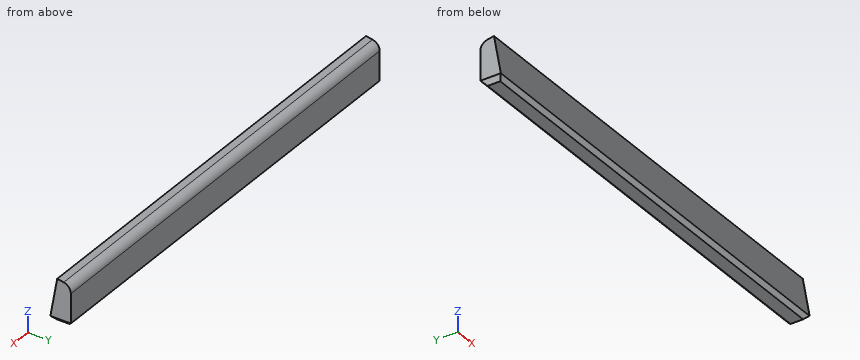
```python
from build123d import *

# Parameters (mm, degrees)
PAD001_DEPTH    = 26
CHAMFER002_SIZE = 0.5
FILLET001_R     = 1


with BuildPart() as part:
    # Sketch002 → Pad001 (new body, symmetric)
    with BuildSketch(Plane.YZ):
        Polygon((0, 0), (-1.575692, 0.277837), (-2.456946, -4.72), (0, -4.72), align=None)
    extrude(amount=PAD001_DEPTH, both=True)

    # Chamfer002
    chamfer002_edges = [part.edges().sort_by_distance(p)[0] for p in [
        (0, -2.456946, -4.72),
        (0, 0, -4.72),
        (-26, -1.228473, -4.72),
        (26, -1.228473, -4.72),
    ]]
    chamfer(chamfer002_edges, length=CHAMFER002_SIZE)

    # Fillet001
    fillet001_edges = [part.edges().sort_by_distance(p)[0] for p in [
        (0, 0, 0),
    ]]
    fillet(fillet001_edges, radius=FILLET001_R)


solid = part.part
```
Verification items for the finished model (mm, model axes). Coordinates: 2 decimals unless noted, no trailing zeros. Write each loop counter-clockwise with the first axis right and the second up, starting at its lowest first coordinate (ties: lowest second). Pieces come first, ordered by that corner, then holes. Notation, with made-up numbers: M 30.5,44.5 L 86.5,44.5 A18 ccw 86.5,67.5 Z; hole C 53,36 d8. An arc over 180 degrees is marked long. Answer as a JSON object with one key per item and string values. Group by question number.
(1) Cross-section at A-A, the plane x = 4. Record the cut outline in (y, z), and give its area (3 significant figures).
(2) Cross-section at B-B, the plane z = -2.35. Record the cut outline in (x, y), and give its area (3 significant figures).
(3) Material ranges on line 1 (Z direction, x = 2, y = -1.2); line 2 (Y direction, x = -22, z = -2.65); line 3 (Z direction, x = -18, y = -0.8), recorded low to high.
Reply:
{
 "1": {"outline": "M -2.37,-4.23 L -1.96,-4.72 L -0.5,-4.72 L 0,-4.22 L 0,-0.84 A1 ccw -0.83,0.15 L -1.58,0.28 Z", "area": "9.47 mm²"},
 "2": {"outline": "M -26,-2.04 L 26,-2.04 L 26,0 L -26,0 Z", "area": "106 mm²"},
 "3": {"line 1": "-4.72 to 0.21", "line 2": "-2.09 to 0", "line 3": "-4.72 to 0.14"}
}
